The listing builds one solid part. Answer for the finished solid, in the listing's coordinates (mm). A direction names the side the tool comes from. Give positions to 0.01 mm unless a question says otherwise; leave off trailing zeros. Write each loop counter-clockwise with the first axis right and the second up, starting at its lowest first coordinate (ties: lowest second). Pieces come first, ordered by that corner, then holes.
```python
from build123d import *

# Parameters (mm, degrees)
SKETCH1_W                                            = 370.50412818
SKETCH1_H                                            = 22.225
BOSS_EXTRUDE1_DEPTH                                  = 38.1
CSK_FOR_M6_HEX_SOCKET_COUNTERSUNK_HEAD_S_D           = 6.4
CSK_FOR_M6_HEX_SOCKET_COUNTERSUNK_HEAD_S_CSINK_D     = 13.5
CSK_FOR_M6_HEX_SOCKET_COUNTERSUNK_HEAD_S_CSINK_ANGLE = 90
SKETCH3_W                                            = 25.4
SKETCH3_H                                            = 25.4
SKETCH3_W_2                                          = 76.2
CUT_EXTRUDE1_DEPTH                                   = 23.225


with BuildPart() as part:
    # Sketch1 → Boss-Extrude1 (new body, symmetric)
    with BuildSketch(Plane(origin=(0, 0, 0), x_dir=(1, 0, 0), z_dir=(0, 1, 0))):
        Rectangle(SKETCH1_W, SKETCH1_H)
    extrude(amount=BOSS_EXTRUDE1_DEPTH, both=True)

    # CSK for M6 Hex Socket Countersunk Head Screw6 (through all)
    with Locations(Plane.XY.offset(11.1125)):
        with Locations((-145.252063961, 16.50746), (-25.252063961, 16.50746), (94.747936039, 16.50746)):
            CounterSinkHole(CSK_FOR_M6_HEX_SOCKET_COUNTERSUNK_HEAD_S_D / 2, CSK_FOR_M6_HEX_SOCKET_COUNTERSUNK_HEAD_S_CSINK_D / 2, counter_sink_angle=CSK_FOR_M6_HEX_SOCKET_COUNTERSUNK_HEAD_S_CSINK_ANGLE)

    # Sketch3 → Cut-Extrude1 (cut, through all)
    with BuildSketch(Plane.XY.offset(11.1125)):
        with Locations((172.55206409, 25.4)):
            Rectangle(SKETCH3_W, SKETCH3_H)
        with Locations((147.15206409, -25.4)):
            Rectangle(SKETCH3_W_2, SKETCH3_H)
    extrude(amount=-CUT_EXTRUDE1_DEPTH, mode=Mode.SUBTRACT)


solid = part.part
```
Item 1: Consider probe 1 along X at (y, z) = (14, 8.25); probe 2 along X at (y, z) = (14, 6); probe 3 along X at (y, z) = (-26.5, 1.25). Determine where each line is inside the solid, lowest interval first.
Conclusion:
probe 1: x = -185.25 to -148.22, -142.28 to -28.22, -22.28 to 91.78, 97.72 to 159.85
probe 2: x = -185.25 to -147.24, -143.26 to -27.24, -23.26 to 92.76, 96.74 to 159.85
probe 3: x = -185.25 to 109.05
Item 2: Which of the six approach directions +Z, -Z, +X, -X, +Y, -Y give full straight-line access (tool end or side, diameter ignored) to faces 1 (the face through (-3, 1, -11.112)), 2 (the face through (147, -12.7, 0)), 3 (the face through (159.852, 25, 0))?
Conclusion:
face 1: -Z, +X, -X, +Y, -Y
face 2: +Z, -Z, +X, -Y
face 3: +Z, -Z, +X, +Y
Item 3: A cutting plane is placed at B-B, the plane y = 29. Give the vertices of the cut face in (x, z), plus the area to 3 significant figures.
Conclusion:
outline: (-185.25, -11.11) - (159.85, -11.11) - (159.85, 11.11) - (-185.25, 11.11) - close
area: 7,670 mm2
Item 4: Determine the mould class of faces 4 (the face through (98.117, 16.656, 7.735)), 5 (the face through (-15, 38.1, 0)), 6 (the face through (185.252, 0, 0)) for opening direction X: pulls with the +X half, pulls with the -X half, needs draft (parallel to the pull), parting line crosses it, or undercut.
Conclusion:
face 4: undercut
face 5: needs draft
face 6: pulls with the +X half
Item 5: A cutting plane is placed at A-A, the plane z = -6. Give the vertices of the cut face in (x, y).
Conclusion:
outline: (-185.25, -38.1) - (109.05, -38.1) - (109.05, -12.7) - (185.25, -12.7) - (185.25, 12.7) - (159.85, 12.7) - (159.85, 38.1) - (-185.25, 38.1) - close; hole circle Ø6.4 at (-145.25, 16.51); hole circle Ø6.4 at (-25.25, 16.51); hole circle Ø6.4 at (94.75, 16.51)
Item 6: Each of these flat-tipped pins is pushed along its axis until it touches: P1, Ø7.5, axis at x = -145.25, y = 16.51, coming from the +Z side; P2, Ø11, axis at x = 141, z = -0.5, coming from the -Y side; P3, Ø6.5, axis at x = 174, z = 4.5, coming from the +Y side; P4, Ø10, axis at x = -25.25, y = 16.51, coming from the -Z side. Where does it stop, or does it pass through?
Conclusion:
P1: stops at z = 8.12
P2: stops at y = -12.7
P3: stops at y = 12.7
P4: stops at z = -11.11
Item 7: A cutting plane is placed at C-C, the plane y = -25.5. Give the vertices of the cut face in (x, z), plus the area to 3 significant figures.
Conclusion:
outline: (-185.25, -11.11) - (109.05, -11.11) - (109.05, 11.11) - (-185.25, 11.11) - close
area: 6,540 mm2
